Verification items for the finished model (mm, model axes). A direction names the side the tool comes from. Give positions to 0.01 mm unless a question says otherwise; leave off trailing zeros. Loops run counter-clockwise (first coordinate to the right, second up) from the corner with the lowest first, then second, coordinate; pieces in that order, holes last. Notation, with made-up numbers: (75.5, 25) - (134.5, 25) arc R22 ccw to (134.5, 51) - close; hole circle Ø1 at (50, -5.75). An arc over 180 degrees is marked (long way). Use one line per item in the form item = value.
```python
from build123d import *

# Parameters (mm, degrees)
LOFTED_BENDS1_DEPTH = 100
SKETCH8_R           = 6.657402664
CUT_EXTRUDE1_DEPTH  = 130


# Read off the part's stored shape, not the designer's step: Lofted Bends1
with BuildPart() as part:
    # Lofted Bends1 outline → Lofted Bends1 (new body)
    with BuildSketch(Plane.XY):
        with BuildLine():
            Line((47.722213143, 0.679631709), (25.978056207, 39.629205506))
            Line((25.978056207, 39.629205506), (24.23175354, 38.654307053))
            Line((24.23175354, 38.654307053), (45.975910476, -0.295266745))
            ThreePointArc((45.975910476, -0.295266745), (46.069270486, -0.664952643), (45.965279678, -1.031790027))
            Line((45.965279678, -1.031790027), (22.732246736, -39.963939806))
            ThreePointArc((22.732246736, -39.963939806), (22.458769362, -40.229634896), (22.089083464, -40.322994907))
            Line((22.089083464, -40.322994907), (-23.24366374, -39.668673062))
            ThreePointArc((-23.24366374, -39.668673062), (-23.610501124, -39.564682253), (-23.876196214, -39.291204879))
            Line((-23.876196214, -39.291204879), (-45.975910476, 0.295266745))
            ThreePointArc((-45.975910476, 0.295266745), (-46.069270486, 0.664952643), (-45.965279678, 1.031790027))
            Line((-45.965279678, 1.031790027), (-22.732246736, 39.963939806))
            ThreePointArc((-22.732246736, 39.963939806), (-22.458769362, 40.229634896), (-22.089083464, 40.322994907))
            Line((-22.089083464, 40.322994907), (22.514315379, 39.679200299))
            Line((22.514315379, 39.679200299), (22.543179886, 41.678991998))
            Line((22.543179886, 41.678991998), (-22.060218957, 42.322786606))
            ThreePointArc((-22.060218957, 42.322786606), (-23.433667815, 41.975937564), (-24.449684896, 40.988833052))
            Line((-24.449684896, 40.988833052), (-47.682717838, 2.056683273))
            ThreePointArc((-47.682717838, 2.056683273), (-48.069062185, 0.69381715), (-47.722213143, -0.679631709))
            Line((-47.722213143, -0.679631709), (-25.622498881, -40.266103333))
            ThreePointArc((-25.622498881, -40.266103333), (-24.63539437, -41.282120414), (-23.272528247, -41.668464761))
            Line((-23.272528247, -41.668464761), (22.060218957, -42.322786606))
            ThreePointArc((22.060218957, -42.322786606), (23.433667815, -41.975937564), (24.449684896, -40.988833052))
            Line((24.449684896, -40.988833052), (47.682717838, -2.056683273))
            ThreePointArc((47.682717838, -2.056683273), (48.069062185, -0.69381715), (47.722213143, 0.679631709))
        make_face()
    extrude(amount=LOFTED_BENDS1_DEPTH)

    # Sketch8 → Cut-Extrude1 (cut)
    with BuildSketch(Plane(origin=(0.606154645, 41.995625683, 0), x_dir=(0.9998958496065499, -0.014432253448298253, 0), z_dir=(0.014432253448298252, 0.9998958496065498, 0))):
        with Locations((0, -17.644210067)):
            Circle(SKETCH8_R)
    extrude(amount=-CUT_EXTRUDE1_DEPTH, mode=Mode.SUBTRACT)


solid = part.part
```
1. Section check B-B, the plane y = -12. Record the cut outline in (x, z).
Result set:
outline = (-41.4, 0) - (-39.11, 0) - (-39.11, 100) - (-41.4, 100) - close; (39.42, 0) - (41.75, 0) - (41.75, 100) - (39.42, 100) - close
2. Scan lines: probe 1 along Y at (x, z) = (2, 74); probe 2 along Y at (x, z) = (-33.5, 21); probe 3 along X at (y, z) = (-6, 59). Record each from-to range of solid material in increasing order.
Result set:
probe_1 = -42.03 to -40.03, 39.98 to 41.98
probe_2 = -26.16 to -22.05, 21.92 to 25.82
probe_3 = -44.75 to -42.46, 43 to 45.33
3. Section check D-D, the plane z = 35.5. Record the cut outline in (x, y), then the cut area to 3 significant figures.
Result set:
outline = (-47.72, -0.68) - (-25.62, -40.27) arc R2.74 ccw to (-23.27, -41.67) - (22.06, -42.32) arc R2.74 ccw to (24.45, -40.99) - (47.68, -2.06) arc R2.74 ccw to (47.72, 0.68) - (25.98, 39.63) - (24.23, 38.65) - (45.98, -0.3) arc R0.74 cw to (45.97, -1.03) - (22.73, -39.96) arc R0.74 cw to (22.09, -40.32) - (-23.24, -39.67) arc R0.74 cw to (-23.88, -39.29) - (-45.98, 0.3) arc R0.74 cw to (-45.97, 1.03) - (-22.73, 39.96) arc R0.74 cw to (-22.09, 40.32) - (22.51, 39.68) - (22.54, 41.68) - (-22.06, 42.32) arc R2.74 ccw to (-24.45, 40.99) - (-47.68, 2.06) arc R2.74 ccw to start
area = 559 mm²
4. Section check A-A, the plane x = -13.5. Record the cut outline in (y, z).
Result set:
outline = (-41.81, 0) - (-39.81, 0) - (-39.81, 100) - (-41.81, 100) - close; (40.2, 0) - (42.2, 0) - (42.2, 100) - (40.2, 100) - close
5. Draft check along Z on faces 1 (the cylindrical face through (-48.07, 0.71, 49.3)), 2 (the flat face through (0, -41, 0)), 3 (the cylindrical face through (-0.275, 41.022, 11.043)). Enter one of: released by +Z, released by -Z, zero draft, split by the parting line, or undercut.
Result set:
face_1 = zero draft
face_2 = released by -Z
face_3 = undercut
6. Depth check by flat-ended pin: pin 1 Ø12 at (x, z) = (3, 18) entering from -Y; pin 2 Ø4 at (x, z) = (-17.5, 33.5) entering from +Y; pin 3 Ø10 at (x, z) = (-35.5, 13.5) entering from +Y; pin 4 Ø1.5 at (x, y) = (-29.5, -24) entering from +Z. Enter the tip coordinate at first touch or a pass-through.
Result set:
pin_1 = -42.13
pin_2 = 42.29
pin_3 = 30.85
pin_4 = through
7. Section check C-C, the plane z = 20.5. State how many separate pieces and enclosed holes the cut face has, then the cut area to 3 significant figures.
Result set:
separate_pieces = 3
enclosed_holes = 0
area = 511 mm²
8. Tool access check on faces 4 (the flat face through (-34.51, 20.23, 49.3)), 5 (the flat face through (-36.827, -20.196, 49.3)). Record the directions out of +Z, -Z, +X, -X, +Y, -Y that give a thin tool (end or side, any length) a straight path to the whole face; none if there is none.
Result set:
face_4 = +Z, -Z
face_5 = +Z, -Z, -X, -Y
